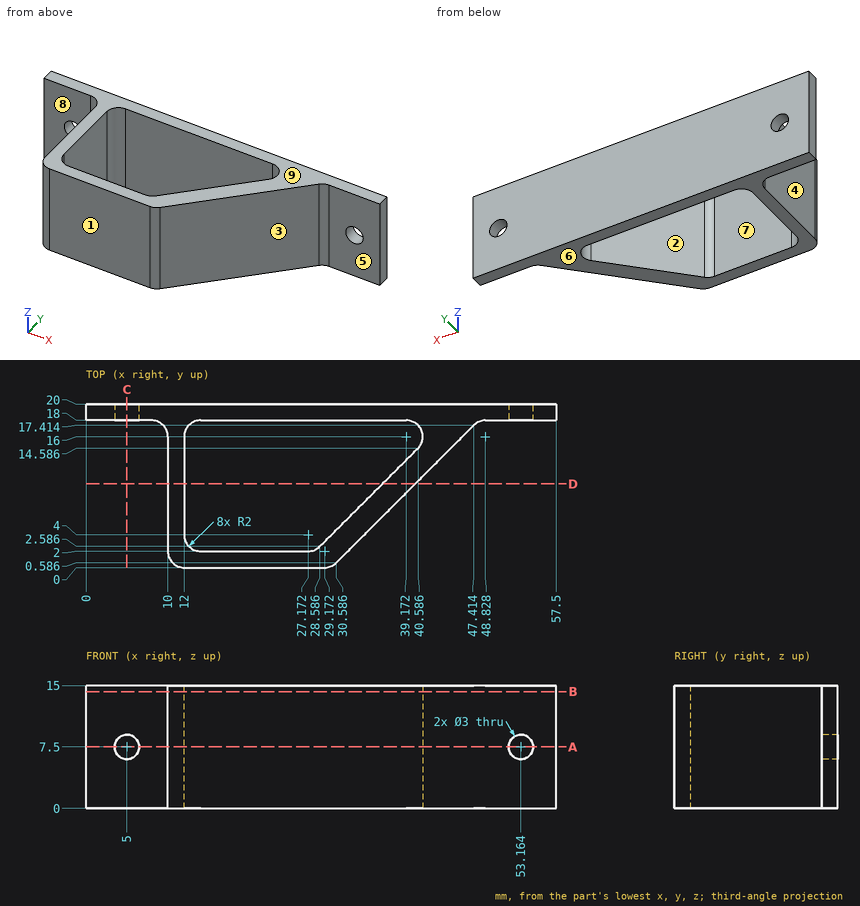
For this review, use the dimensioned drawing (mm, ordinates from the lowest corner) and the shaded views. A direction names the side the tool comes from. Round coordinates to 2 decimals unless told otherwise and drop trailing zeros. Order: outer loops, then holes, each group sorted by start corner. A loop starts at its lowest first (then second) coordinate and runs counter-clockwise, first axis right, second up. Notation, with made-up numbers: M -35,72.5 L 4,72.5 A21 cw 4,88.5 Z; hole C 76.25,-12 d6. An arc over 180 degrees is marked long. Use a Markdown table: item, result.
1) Consider section D-D (y = 10.25). Write out the cut boundary in (x, z).
Report:
| item | result |
|---|---|
| outline | M 10,0 L 12,0 L 12,15 L 10,15 Z; M 36.25,0 L 40.25,0 L 40.25,15 L 36.25,15 Z |
2) Wall thickness on line 1 along X through (y, z) = (19.5, 7.5) (1 decimal); line 2 along Y through (x, z) = (25, 3); line 3 along Z through (x, y) = (5, 18.85): over which ranges is each line inside the solid? List them lowest first. Write a range as [from, to].
Report:
| item | result |
|---|---|
| line 1 | [0, 3.5], [6.5, 51.7], [54.7, 57.5] |
| line 2 | [0, 2], [18, 20] |
| line 3 | [0, 6], [9, 15] |
3) Insertion check: pin 1 (1.5 mm diameter, centred on x = 18.5, y = 17.5, fed in from +Z); pin 2 (2.5 mm diameter, centred on x = 4.5, z = 10, fed in from -Y); pin 3 (8 mm diameter, centred on y = 10, z = 6, fed in from -X); pin 4 (5 mm diameter, centred on y = 13.5, z = 4.5, fed in from +X). Each pin has a flat end and moves straight along its axis. Give the tip position at first contact, or say it passes through.
Report:
| item | result |
|---|---|
| pin 1 | z = 15 |
| pin 2 | y = 18 |
| pin 3 | x = 10 |
| pin 4 | x = 46 |
4) Draft analysis for pull direction X (two halves, no side actions). For the marked faces 1, 2, 3 and 4, state which applies: released by +X, released by -X, zero draft, split by the parting line, or undercut.
Report:
| item | result |
|---|---|
| face 1 | zero draft |
| face 2 | undercut |
| face 3 | released by +X |
| face 4 | released by -X |
5) Consider section A-A (z = 7.5). Write out the cut boundary in (x, y) (1 decimal).
Report:
| item | result |
|---|---|
| outline | M 0,18 L 3.5,18 L 3.5,20 L 0,20 Z; M 6.5,18 L 8,18 A2 cw 10,16 L 10,2 A2 ccw 12,0 L 29.2,0 A2 ccw 30.6,0.6 L 47.4,17.4 A2 cw 48.8,18 L 51.7,18 L 51.7,20 L 6.5,20 Z; M 54.7,18 L 57.5,18 L 57.5,20 L 54.7,20 Z; hole M 12,4 A2 ccw 14,2 L 27.2,2 A2 ccw 28.6,2.6 L 40.6,14.6 A2 ccw 39.2,18 L 14,18 A2 ccw 12,16 Z |
6) Tool access review of the marked faces 5, 6, 7, 8 and 9: name each direction out of +Z, -Z, +X, -X, +Y, -Y from which nothing blocks a thin tool from reaching the whole face with its end or side.
Report:
| item | result |
|---|---|
| face 5 | +Z, -Z, +X, -Y |
| face 6 | -Z, +X, -X, +Y, -Y |
| face 7 | +Z, -Z |
| face 8 | +Z, -Z, -X, -Y |
| face 9 | +Z, +X, -X, +Y, -Y |
7) Consider section C-C (x = 5). Write out the cut boundary in (y, z).
Report:
| item | result |
|---|---|
| outline | M 18,0 L 20,0 L 20,6 L 18,6 Z; M 18,9 L 20,9 L 20,15 L 18,15 Z |
8) Consider section B-B (z = 14.25). Write out the cut boundary in (x, y) (1 decimal).
Report:
| item | result |
|---|---|
| outline | M 0,18 L 8,18 A2 cw 10,16 L 10,2 A2 ccw 12,0 L 29.2,0 A2 ccw 30.6,0.6 L 47.4,17.4 A2 cw 48.8,18 L 57.5,18 L 57.5,20 L 0,20 Z; hole M 12,4 A2 ccw 14,2 L 27.2,2 A2 ccw 28.6,2.6 L 40.6,14.6 A2 ccw 39.2,18 L 14,18 A2 ccw 12,16 Z |
